from build123d import *

# Parameters (mm, degrees)
SKETCH1_R               = 6.35
BOSS_EXTRUDE1_DEPTH     = 95.8088
SKETCH4_R               = 3.175
CUT_EXTRUDE2_DEPTH      = 7.35
CUT_EXTRUDE2_DEPTH_BACK = 7.35
SKETCH5_R               = 19.05
BOSS_EXTRUDE2_DEPTH     = 2.54
SKETCH6_R               = 19.05
BOSS_EXTRUDE3_DEPTH     = 2.54
CUT_EXTRUDE4_DEPTH      = 27.94
CUT_EXTRUDE5_DEPTH      = 27.94


with BuildPart() as part:
    # Sketch1 → Boss-Extrude1 (new body)
    with BuildSketch(Plane.XY):
        Circle(SKETCH1_R)
    extrude(amount=BOSS_EXTRUDE1_DEPTH)

    # Sketch4 → Cut-Extrude2 (cut, two sides)
    with BuildSketch(Plane(origin=(0, 0, 0), x_dir=(1, 0, 0), z_dir=(0, 1, 0))) as cut_extrude2_sk:
        with Locations((0, -64.0588)):
            Circle(SKETCH4_R)
        with Locations((0, -31.75)):
            Circle(SKETCH4_R)
    extrude(amount=CUT_EXTRUDE2_DEPTH, mode=Mode.SUBTRACT)
    extrude(cut_extrude2_sk.sketch, amount=-CUT_EXTRUDE2_DEPTH_BACK, mode=Mode.SUBTRACT)

    # Sketch5 → Boss-Extrude2 (add)
    with BuildSketch(Plane.XY.offset(57.7088)):
        Circle(SKETCH5_R)
    extrude(amount=-BOSS_EXTRUDE2_DEPTH)

    # Sketch6 → Boss-Extrude3 (add)
    with BuildSketch(Plane(origin=(0, 0, 38.1), x_dir=(-1, 0, 0), z_dir=(0, 0, -1))):
        Circle(SKETCH6_R)
    extrude(amount=-BOSS_EXTRUDE3_DEPTH)

    # Sketch2 → Cut-Extrude4 (cut)
    with BuildSketch(Plane.XY.offset(95.8088)):
        with BuildLine():
            Line((-1.992888597, -2.5527), (1.992888597, -2.5527))
            ThreePointArc((1.992888597, -2.5527), (0, 3.2385), (-1.992888597, -2.5527))
        make_face()
    extrude(amount=-CUT_EXTRUDE4_DEPTH, mode=Mode.SUBTRACT)

    # Sketch7 → Cut-Extrude5 (cut)
    with BuildSketch(Plane(origin=(0, 0, 0), x_dir=(-1, 0, 0), z_dir=(0, 0, -1))):
        with BuildLine():
            Line((-2.5527, 1.992888597), (-2.5527, -1.992888597))
            ThreePointArc((-2.5527, -1.992888597), (1.053793931, -3.06225417), (3.2385, 0))
            ThreePointArc((3.2385, 0), (1.053793931, 3.06225417), (-2.5527, 1.992888597))
        make_face()
    extrude(amount=-CUT_EXTRUDE5_DEPTH, mode=Mode.SUBTRACT)


solid = part.part
CAD build for the part. Positions are in the model's coordinates, mm. A direction names the side the tool comes from. Give positions to 0.01 mm unless a question says otherwise; leave off trailing zeros. Write each loop counter-clockwise with the first axis right and the second up, starting at its lowest first coordinate (ties: lowest second). Pieces come first, ordered by that corner, then holes. Notation, with made-up numbers: (71.25, -20.75) -> (101.25, -20.75) arc R14 ccw to (101.25, -2.75) -> close; hole circle Ø4 at (89.5, -23). An arc over 180 degrees is marked (long way). Return JSON: item names as keys, results as strings.
Item 1: Tool access for faces 1 (the flat face through (0, 0, 27.94)), 2 (the cylindrical face through (-15.12, -11.59, 56.46)), 3 (the flat face through (5, 5, 40.64)), 4 (the flat face through (0, 0, 67.869)): list every direction of +Z, -Z, +X, -X, +Y, -Y with a clear straight run to the whole face (end or side of a thin tool).
Answer below:
{"face 1": "-Z", "face 2": "+Z, -Z", "face 3": "none", "face 4": "+Z"}
Item 2: Drill centre lines: probe 1 along Z at (x, y) = (0, -4) (3 decimals); probe 2 along Z at (x, y) = (5, -15.5); probe 3 along Y at (x, z) = (0, 75). Where is each one in solid material? Low to high.
Answer below:
{"probe 1": "z = 0 to 28.575, 34.925 to 60.884, 67.234 to 95.809", "probe 2": "z = 38.1 to 40.64, 55.17 to 57.71", "probe 3": "y = -6.35 to -2.55, 3.24 to 6.35"}
Item 3: Band-saw the part on A-A (x = -17). List the corners of the cut face in (y, z).
Answer below:
{"outline": "(-8.6, 38.1) -> (8.6, 38.1) -> (8.6, 40.64) -> (-8.6, 40.64) -> close; (-8.6, 55.17) -> (8.6, 55.17) -> (8.6, 57.71) -> (-8.6, 57.71) -> close"}
Item 4: Band-saw the part on B-B (y = 12). List the corners of the cut face in (x, z).
Answer below:
{"outline": "(-14.8, 38.1) -> (14.8, 38.1) -> (14.8, 40.64) -> (-14.8, 40.64) -> close; (-14.8, 55.17) -> (14.8, 55.17) -> (14.8, 57.71) -> (-14.8, 57.71) -> close"}
Item 5: Band-saw the part on C-C (z = 82). List the corners of the cut face in (x, y), then the cut area to 3 significant figures.
Answer below:
{"outline": "circle Ø12.7 at (0, 0); hole (-1.99, -2.55) -> (1.99, -2.55) arc R3.24 ccw (long way) to start", "area": "95.6 mm2"}
Item 6: Drop flat-ended pins along their axis: pin 1 (1.2 mm diameter, centred on y = -0.5, z = 12.5, fed in from -X); pin 2 (1.5 mm diameter, centred on y = 2, z = 54.5, fed in from -X); pin 3 (5 mm diameter, centred on x = 2.5, z = 75, fed in from -Y); pin 4 (5 mm diameter, centred on x = 0, z = 64.06, fed in from +Y). Give the stop position or say it passes through.
Answer below:
{"pin 1": "stops at x = -6.35", "pin 2": "stops at x = -18.98", "pin 3": "stops at y = -6.35", "pin 4": "passes through"}
Item 7: Band-saw the part on D-D (x = 0). Give the number of separate pieces and of enclosed holes in the cut face, then the cut area to 3 significant figures.
Answer below:
{"separate pieces": "3", "enclosed holes": "0", "area": "842 mm2"}
Item 8: Two-plate mould, pull along X, no slides. Class faces 5 (the flat face through (0, -2.553, 82)), 6 (the flat face through (-5, 5, 55.169)), 7 (the cylindrical face through (-1.38, -6.2, 47.8)): +X half, -X half, draft (parallel to the pull), parting line (faces both ways), or undercut.
Answer below:
{"face 5": "undercut", "face 6": "draft", "face 7": "parting line"}
